Input: part model. Units: mm. Frame: model coordinates. Give positions to 0.01 mm unless a question says otherwise; leave off trailing zeros. Order: outer loops, then holes, each group sorted by start corner. A loop starts at its lowest first (then second) coordinate and runs counter-clockwise, first axis right, second up. Notation, with made-up numbers: (3.5, 16.5) - (48.5, 16.5) arc R8 ccw to (48.5, 21.5) - close; hole circle Ø1 at (27.5, 73.25). An arc over 180 degrees is marked (long way). Answer in a Markdown table with one row per item. Add a question column.
Autodesk Inventor part; units mm, degrees
ref_plane "YZ Plane" through (0, 0, 0) normal (1, 0, 0) x (0, 1, 0)
ref_plane "XZ Plane" through (0, 0, 0) normal (0, 1, 0) x (-1, 0, 0)
ref_plane "XY Plane" through (0, 0, 0) normal (0, 0, 1) x (1, 0, 0)
sketch "Sketch1" plane through (0, 0, 0) normal (0, 1, 0) x (-1, 0, 0)
  line L0 (0, 0) -> (-57.5, 0)
  line L1 (-57.5, 0) -> (-57.5, -9.525)
  line L2 (-57.5, -9.525) -> (0, -9.525)
  line L3 (0, -9.525) -> (0, 0)
  line L4 (0, -4.7625) -> (-57.5, -4.7625) construction
  circle A0 centre (-7.493, -4.7625) radius 1.5
  circle A1 centre (-53.5, -4.7625) radius 1.5
  circle A2 centre (-30.4927, -4.7625) radius 1.5
  dimension "d0" = 9.525
  dimension "d1" = 57.5
  dimension "d2" = 3
  dimension "d3" = 7.493
  dimension "d4" = 4
  dimension "d14" = 22.9997
  dimension "d15" = 23.0073
extrude "Extrusion1" add sketch "Sketch1" along normal blind 18 contours L3 L2 L1 L0 | A0 | A1 | A2
hole "Hole1" at (53.5, 0, -4.7625) at (7.493, 0, -4.7625) at (30.4927, 0, -4.7625) direction (0, 1, 0) diameter 3.4036 end through all
properties part number "Drive Frame Spacing Block" material "Aluminum 6061"
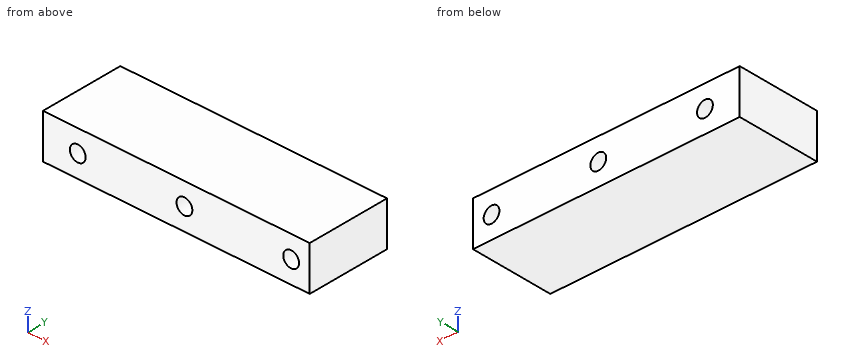
Q1. Line query: probe 1 along X at (y, z) = (5, -4.75); probe 2 along X at (y, z) = (2, -6); probe 3 along Z at (x, y) = (53.5, 3.75) (3 decimals). Output: solid intervals per line, ascending.
Q2. Contact query for flat-ended pins moving along their axis: P1, Ø5.5, axis at x = 7.49, z = -4.76, coming from the -Y side; P2, Ø2.5, axis at x = 30.49, z = -4.76, coming from the -Y side. Output: stop coordinate, or through.
Q3. Section C-C, the plane z = -5.5. Return loops of the section in (x, y).
Q4. Section B-B, the plane y = 9.25. Return loops of the section in (x, z) (1 decimal).
Q5. Section A-A, the plane x = 53.5. Return loops of the section in (y, z) (3 decimals), then the cut area to 3 significant figures.
Computed:
| question | item | result |
|---|---|---|
| 1 | probe 1 | x = 0 to 5.79, 9.19 to 28.79, 32.19 to 51.8, 55.2 to 57.5 |
| 1 | probe 2 | x = 0 to 6.32, 8.66 to 29.32, 31.66 to 52.33, 54.67 to 57.5 |
| 1 | probe 3 | z = -9.525 to -6.464, -3.061 to 0 |
| 2 | P1 | stops at y = 0 |
| 2 | P2 | passes through |
| 3 | outline | (0, 0) - (5.96, 0) - (5.96, 18) - (0, 18) - close; (9.03, 0) - (28.96, 0) - (28.96, 18) - (9.03, 18) - close; (32.03, 0) - (51.97, 0) - (51.97, 18) - (32.03, 18) - close; (55.03, 0) - (57.5, 0) - (57.5, 18) - (55.03, 18) - close |
| 4 | outline | (0, -9.5) - (57.5, -9.5) - (57.5, 0) - (0, 0) - close; hole circle Ø3.4 at (7.5, -4.8); hole circle Ø3.4 at (30.5, -4.8); hole circle Ø3.4 at (53.5, -4.8) |
| 5 | outline | (0, -9.525) - (18, -9.525) - (18, -6.464) - (0, -6.464) - close; (0, -3.061) - (18, -3.061) - (18, 0) - (0, 0) - close |
| 5 | area | 110 mm^2 |
